from build123d import *

# Parameters (mm, degrees)
ESQUISSE1_W             = 159
ESQUISSE1_H             = 104
BOSS_EXTRU_1_DEPTH      = 6
ESQUISSE2_W             = 24
ESQUISSE2_H             = 6
ESQUISSE2_W_2           = 45
ESQUISSE2_W_3           = 30
ENL_V_MAT_EXTRU_1_DEPTH = 191.086822268
ESQUISSE3_R             = 1.5
ENL_V_MAT_EXTRU_2_DEPTH = 191.086822268
ESQUISSE4_R             = 2.995
ENL_V_MAT_EXTRU_3_DEPTH = 3
ESQUISSE5_W             = 30
ESQUISSE5_H             = 6
BOSS_EXTRU_2_DEPTH      = 6
ESQUISSE6_W             = 30
ESQUISSE6_H             = 6
ENL_V_MAT_EXTRU_4_DEPTH = 3


with BuildPart() as part:
    # Esquisse1 → Boss.-Extru.1 (new body)
    with BuildSketch(Plane.XY):
        with Locations((-79.5, 52)):
            Rectangle(ESQUISSE1_W, ESQUISSE1_H)
    extrude(amount=BOSS_EXTRU_1_DEPTH)

    # Esquisse2 → Enlèv. mat.-Extru.1 (cut, through all)
    with BuildSketch(Plane.XY.offset(6)):
        with Locations((-147, 101)):
            Rectangle(ESQUISSE2_W, ESQUISSE2_H)
        with Locations((-22.5, 101)):
            Rectangle(ESQUISSE2_W_2, ESQUISSE2_H)
        with Locations((-90, 101)):
            Rectangle(ESQUISSE2_W_3, ESQUISSE2_H)
    extrude(amount=-ENL_V_MAT_EXTRU_1_DEPTH, mode=Mode.SUBTRACT)

    # Esquisse3 → Enlèv. mat.-Extru.2 (cut, through all)
    with BuildSketch(Plane.XY.offset(6)):
        with Locations((-128, 101)):
            Circle(ESQUISSE3_R)
        with Locations((-112, 101)):
            Circle(ESQUISSE3_R)
        with Locations((-68, 101)):
            Circle(ESQUISSE3_R)
        with Locations((-52, 101)):
            Circle(ESQUISSE3_R)
    extrude(amount=-ENL_V_MAT_EXTRU_2_DEPTH, mode=Mode.SUBTRACT)

    # Esquisse4 → Enlèv. mat.-Extru.3 (cut)
    with BuildSketch(Plane.XY.offset(6)):
        with Locations((-128, 101)):
            Circle(ESQUISSE4_R)
        with Locations((-112, 101)):
            Circle(ESQUISSE4_R)
        with Locations((-68, 101)):
            Circle(ESQUISSE4_R)
        with Locations((-52, 101)):
            Circle(ESQUISSE4_R)
    extrude(amount=-ENL_V_MAT_EXTRU_3_DEPTH, mode=Mode.SUBTRACT)

    # Esquisse5 → Boss.-Extru.2 (add)
    with BuildSketch(Plane.XZ):
        with Locations((-84, 3)):
            Rectangle(ESQUISSE5_W, ESQUISSE5_H)
    extrude(amount=BOSS_EXTRU_2_DEPTH)

    # Esquisse6 → Enlèv. mat.-Extru.4 (cut)
    with BuildSketch(Plane(origin=(0, 0, 0), x_dir=(-1, 0, 0), z_dir=(0, 0, -1))):
        with Locations((84, -3)):
            Rectangle(ESQUISSE6_W, ESQUISSE6_H)
    extrude(amount=-ENL_V_MAT_EXTRU_4_DEPTH, mode=Mode.SUBTRACT)


solid = part.part
The listing builds one solid part. Answer for the finished solid, in the listing's coordinates (mm). A direction names the side the tool comes from. Round coordinates to 2 decimals unless told otherwise and drop trailing zeros. Write each loop counter-clockwise with the first axis right and the second up, starting at its lowest first coordinate (ties: lowest second). Pieces come first, ordered by that corner, then holes. Notation, with made-up numbers: M 72.25,3.5 L 92.25,3.5 A19 ccw 92.25,22.5 Z; hole C -37.5,89.5 d2. An arc over 180 degrees is marked long. Write each question's results on one line, items separated by ' | '. Start each with the question number.
Item 1: Find section C-C on x = -122. Write down the section's boundary in (y, z), and give its area (3 significant figures).
Item 2: Find section A-A on z = 3.95. Write down the section's boundary in (x, y) (3 decimals).
Item 3: Find section D-D on x = -40.5. Write down the section's boundary in (y, z), and give its area (3 significant figures).
Item 4: Given pin 1 Ø1.8 at (x, y) = (-111, 101.5) entering from +Z; pin 2 Ø1 at (x, z) = (-26, 1.5) entering from -Y; pin 3 Ø3 at (y, z) = (101, 1.5) entering from +X; pin 4 Ø2.5 at (x, y) = (-112, 101) entering from +Z, each flat-ended and moving along its own axis, determine where each tip first touches the part or whether it passes through.
Item 5: Straight lines are drawn through the part: probe 1 along Y at (x, z) = (-112, 2.4); probe 2 along X at (y, z) = (99, 1.45); probe 3 along Y at (x, z) = (-58.5, 5.4). For each, find the intervals that lie inside material, in ascending order.
Item 6: Find section B-B on x = -89. Write down the section's boundary in (y, z), and give its area (3 significant figures).
Item 7: Which of the six approach directions +Z, -Z, +X, -X, +Y, -Y give full straight-line access (tool end or side, diameter ignored) to faces 1 (the flat face through (-105, 101, 3)), 2 (the cylindrical face through (-113.11, 102.01, 1.52)), 3 (the cylindrical face through (-49.233, 99.853, 4.521)), 4 (the flat face through (-23, 98, 3))?
Item 8: The mould has two halves that part along X. Classify faces 5 (the cylindrical face through (-70.992, 101.132, 4.521)), 6 (the cylindrical face through (-67.194, 102.265, 1.521)), 7 (the flat face through (-147, 98, 3)), 8 (the flat face through (-135, 101, 3)): +X half, -X half, draft (parallel to the pull), parting line (faces both ways), or undercut.
Answer block:
1) outline: M 0,0 L 104,0 L 104,6 L 0,6 Z | area: 624 mm²
2) outline: M -159,0 L -99,0 L -99,-6 L -69,-6 L -69,0 L 0,0 L 0,98 L -45,98 L -45,104 L -75,104 L -75,98 L -105,98 L -105,104 L -135,104 L -135,98 L -159,98 Z; hole C -128,101 d5.99; hole C -112,101 d5.99; hole C -68,101 d5.99; hole C -52,101 d5.99
3) outline: M 0,0 L 98,0 L 98,6 L 0,6 Z | area: 588 mm²
4) pin 1: stops at z = 3 | pin 2: stops at y = 0 | pin 3: stops at x = -45 | pin 4: passes through
5) probe 1: y = 0 to 99.5, 102.5 to 104 | probe 2: x = -135 to -105, -75 to -45 | probe 3: y = 0 to 104
6) outline: M -6,3 L 0,3 L 0,0 L 98,0 L 98,6 L -6,6 Z | area: 606 mm²
7) face 1: +Z, -Z, +Y | face 2: +Z, -Z | face 3: +Z | face 4: +Z, -Z, +X, +Y
8) face 5: undercut | face 6: undercut | face 7: draft | face 8: -X half
